from build123d import *

# Parameters (mm, degrees)
SKETCH_1_W                    = 45
SKETCH_1_H                    = 26
BOSS_EXTRUDE1_DEPTH           = 17
SKETCH_W                      = 48
SKETCH_H                      = 28.5
BOSS_EXTRUDE2_DEPTH           = 2.2
SKETCH_3_W                    = 36
SKETCH_3_H                    = 16.5
CUT_EXTRUDE1_DEPTH            = 3
CHAMFER_1_SIZE                = 3
CHAMFER_1_SIZE2               = 1.732050808
SKETCH_4_R                    = 0.625
BOSS_EXTRUDE3_DEPTH           = 0.1
ROUNDING_1_R                  = 1.05
LINEAR_ARRAY1_COUNT           = 3
LINEAR_ARRAY1_PITCH           = 12.5
ROUNDING_1_OF_LINEAR_ARRAY1_R = 1.05


with BuildPart() as part:
    # sketch 1 → Boss-Extrude1 (new body)
    with BuildSketch(Plane.XY):
        Rectangle(SKETCH_1_W, SKETCH_1_H)
    extrude(amount=BOSS_EXTRUDE1_DEPTH)

    # sketch → Boss-Extrude2 (add)
    with BuildSketch(Plane.XY.offset(17)):
        Rectangle(SKETCH_W, SKETCH_H)
    extrude(amount=BOSS_EXTRUDE2_DEPTH)

    # sketch 3 → Cut-Extrude1 (cut)
    with BuildSketch(Plane.XY.offset(19.2)):
        Rectangle(SKETCH_3_W, SKETCH_3_H)
    extrude(amount=-CUT_EXTRUDE1_DEPTH, mode=Mode.SUBTRACT)

    # chamfer 1
    chamfer_1_edges = [part.edges().sort_by_distance(p)[0] for p in [
        (-18, 0, 19.2),
        (0, -8.25, 19.2),
        (18, 0, 19.2),
        (0, 8.25, 19.2),
    ]]
    chamfer_1_side = [part.faces().sort_by_distance(p)[0] for p in [
        (0, -13.691766178, 19.2),
    ]]
    chamfer(chamfer_1_edges, length=CHAMFER_1_SIZE, length2=CHAMFER_1_SIZE2, reference=chamfer_1_side[0])

    # sketch 4 → Boss-Extrude3 (add)
    with BuildSketch(Plane.XY.offset(16.2)):
        with Locations((-8.310233245, -6.125)):
            Circle(SKETCH_4_R)
        Polygon((-17.8, -6.75), (-16.531988477, -6.75), (-15.515440373, -0.783304607), (-16.049974064, -0.15), (-16.675555556, -0.15), align=None)
        Polygon((-9.68472625, -6.75), (-8.560281805, -0.15), (-9.077616658, -0.15), (-9.954369729, -0.890013653), (-10.952737773, -6.75), align=None)
        Polygon((-15.5, 6.75), (-14.231988477, 6.75), (-15.236353449, 0.854814294), (-16.071403038, 0.15), (-16.624444444, 0.15), align=None)
        Polygon((-8.509170694, 0.15), (-9.099045632, 0.15), (-9.66328895, 0.818503966), (-8.652737773, 6.75), (-7.38472625, 6.75), align=None)
        Polygon((-15.784003603, 0), (-15.04351636, 0.625), (-9.892540373, 0.625), (-9.365016093, 0), (-10.105503336, -0.625), (-15.256479323, -0.625), align=None)
        Polygon((-13.927665711, 6.75), (-14.140628674, 5.5), (-9.170023502, 5.5), (-8.957060539, 6.75), align=None)
        Polygon((-16.227665711, -6.75), (-16.014702748, -5.5), (-11.044097576, -5.5), (-11.257060539, -6.75), align=None)
    boss_extrude3 = extrude(amount=BOSS_EXTRUDE3_DEPTH)

    # rounding 1
    rounding_1_edges = [part.edges().sort_by_distance(p)[0] for p in [
        (-17.8, -6.75, 16.25),
        (-9.68472625, -6.75, 16.25),
        (-7.38472625, 6.75, 16.25),
        (-15.5, 6.75, 16.25),
    ]]
    fillet(rounding_1_edges, radius=ROUNDING_1_R)

    # Linear array1: Boss-Extrude3 ×3
    with Locations(*[(i * LINEAR_ARRAY1_PITCH, 0, 0) for i in range(1, LINEAR_ARRAY1_COUNT)]):
        add(boss_extrude3)

    # rounding 1 of Linear array1
    rounding_1_of_linear_array1_edges = [part.edges().sort_by_distance(p)[0] for p in [
        (-5.3, -6.75, 16.25),
        (2.81527375, -6.75, 16.25),
        (5.11527375, 6.75, 16.25),
        (-3, 6.75, 16.25),
        (7.2, -6.75, 16.25),
        (15.31527375, -6.75, 16.25),
        (17.61527375, 6.75, 16.25),
        (9.5, 6.75, 16.25),
    ]]
    fillet(rounding_1_of_linear_array1_edges, radius=ROUNDING_1_OF_LINEAR_ARRAY1_R)


solid = part.part
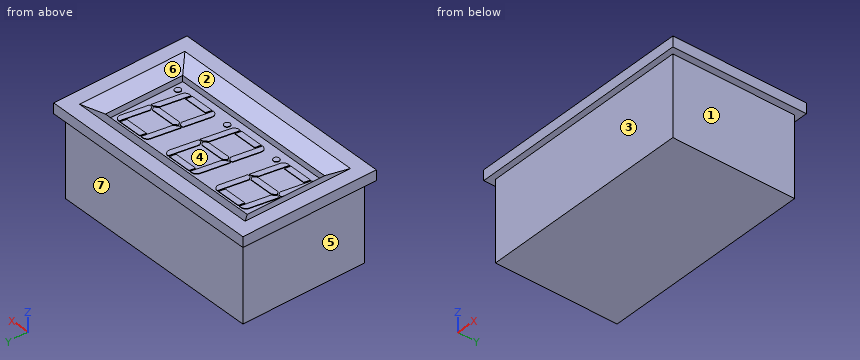
Can you work these out from the model? Positions are in its coordinate system, mm. Face numbers are marked on the shaded views. A direction names the side the tool comes from. Give positions to 0.01 mm unless a question says otherwise; leave off trailing zeros. Loops run counter-clockwise (first coordinate to the right, second up) from the corner with the lowest first, then second, coordinate; pieces in that order, holes last. Notation, with made-up numbers: (55.5, -9.75) -> (89.5, -9.75) arc R17 ccw to (89.5, 11.25) -> close; hole circle Ø4 at (9.5, 52). An arc over 180 degrees is marked (long way). Return JSON: item names as keys, results as strings.
Q1. I want a section at C-C, the plane z = 9. List the corners of the cut face in (x, y) for me, then the cut area to 3 significant figures.
Checks:
{"outline": "(-22.5, -13) -> (22.5, -13) -> (22.5, 13) -> (-22.5, 13) -> close", "area": "1,170 mm2"}
Q2. I want a section at A-A, the plane x = 0.5. List the corners of the cut face in (y, z) for me (3 decimals), then the cut area to 3 significant figures.
Checks:
{"outline": "(-14.25, 17) -> (-13, 17) -> (-13, 0) -> (13, 0) -> (13, 17) -> (14.25, 17) -> (14.25, 19.2) -> (11.25, 19.2) -> (8.25, 17.468) -> (8.25, 16.2) -> (6.75, 16.2) -> (6.75, 16.3) -> (5.5, 16.3) -> (5.5, 16.2) -> (0.625, 16.2) -> (0.625, 16.3) -> (-0.625, 16.3) -> (-0.625, 16.2) -> (-5.5, 16.2) -> (-5.5, 16.3) -> (-6.75, 16.3) -> (-6.75, 16.2) -> (-8.25, 16.2) -> (-8.25, 17.468) -> (-11.25, 19.2) -> (-14.25, 19.2) -> close", "area": "450 mm2"}
Q3. I want a section at D-D, the plane x = 20. List the corners of the cut face in (y, z) for me.
Checks:
{"outline": "(-14.25, 17) -> (-13, 17) -> (-13, 0) -> (13, 0) -> (13, 17) -> (14.25, 17) -> (14.25, 19.2) -> (11.25, 19.2) -> (10.25, 18.62) -> (-10.25, 18.62) -> (-11.25, 19.2) -> (-14.25, 19.2) -> close"}
Q4. We'd pull the mould along X, two halves only. Please class the marked faces 4, 5, 6 and 7: released by +X, released by -X, zero draft, split by the parting line, or undercut.
Checks:
{"face 4": "undercut", "face 5": "released by -X", "face 6": "undercut", "face 7": "zero draft"}
Q5. On a 3-axis mill with a long thin cutter (end or side, diameter ignored), from which of +Z, -Z, +X, -X, +Y, -Y can I reach the whole of each face in a straight line? I mean the marked faces 1, 2 and 3. Say none if no direction works.
Checks:
{"face 1": "-Z, +X, +Y, -Y", "face 2": "+Z", "face 3": "-Z, +X, -X, -Y"}
Q6. I need wall thicknesses on probe 1 along Y at (x, z) = (-21.5, 14.5); probe 2 along X at (y, z) = (11.75, 15.25); probe 3 along Y at (x, z) = (-15, 17.25). Which ranges of each line are inside material? Lowest first, please.
Checks:
{"probe 1": "y = -13 to 13", "probe 2": "x = -22.5 to 22.5", "probe 3": "y = -14.25 to -8.25, 8.25 to 14.25"}
Q7. I want a section at B-B, the plane y = 9.5. List the corners of the cut face in (x, z) for me, then the cut area to 3 significant figures.
Checks:
{"outline": "(-24, 17) -> (-22.5, 17) -> (-22.5, 0) -> (22.5, 0) -> (22.5, 17) -> (24, 17) -> (24, 19.2) -> (21, 19.2) -> (19.25, 18.19) -> (-19.25, 18.19) -> (-21, 19.2) -> (-24, 19.2) -> close", "area": "830 mm2"}
Q8. For pin 1 Ø6 at (x, y) = (-6.5, 8) entering from -Z; pin 2 Ø1 at (y, z) = (2, 5.5) entering from +X; pin 3 Ø5 at (x, z) = (19, 11) entering from +Y; pin 4 Ø0.7 at (x, y) = (-3, 5) entering from +Z, each with a flat end and sliding along its axis, tell me the tip position at first contact or that it passes through.
Checks:
{"pin 1": "stops at z = 0", "pin 2": "stops at x = 22.5", "pin 3": "stops at y = 13", "pin 4": "stops at z = 16.3"}
